from build123d import *

# Parameters (mm, degrees)
RESSALTO_EXTRUS_O1_DEPTH = 56
FILETE1_R                = 0.5
ESBO_O2_R                = 0.751353762
CORTE_EXTRUS_O1_DEPTH    = 57


with BuildPart() as part:
    # Esboço1 → Ressalto-extrusão1 (new body)
    with BuildSketch(Plane.XZ.offset(30)):
        Polygon((-1.443375673, -2.5), (1.443375673, -2.5), (2.886751346, 0), (1.443375673, 2.5), (-1.443375673, 2.5), (-2.886751346, 0), align=None)
    extrude(amount=-RESSALTO_EXTRUS_O1_DEPTH)

    # Filete1
    filete1_edges = [part.edges().sort_by_distance(p)[0] for p in [
        (2.165063509, 26, -1.25),
        (2.165063509, 26, 1.25),
        (0, 26, 2.5),
        (-2.165063509, 26, 1.25),
        (-2.165063509, 26, -1.25),
        (-2.165063509, -30, 1.25),
        (0, -30, 2.5),
        (2.165063509, -30, 1.25),
        (2.165063509, -30, -1.25),
        (0, -30, -2.5),
        (-2.165063509, -30, -1.25),
        (0, 26, -2.5),
    ]]
    fillet(filete1_edges, radius=FILETE1_R)

    # Esboço2 → Corte-extrusão1 (cut, through all)
    with BuildSketch(Plane.XZ.offset(30)):
        Circle(ESBO_O2_R)
    extrude(amount=-CORTE_EXTRUS_O1_DEPTH, mode=Mode.SUBTRACT)


solid = part.part
CAD build for the part. Positions are in the model's coordinates, mm. Round coordinates to 2 decimals unless told otherwise and drop trailing zeros. Loops run counter-clockwise (first coordinate to the right, second up) from the corner with the lowest first, then second, coordinate; pieces in that order, holes last. Notation, with made-up numbers: M 68,27.25 L 90,27.25 A34 ccw 90,58.25 Z; hole C 16,72 d9. An arc over 180 degrees is marked long. One line per question, with ' | ' between items. Start each with the question number.
Item 1: Cut at A-A, the plane y = 21. Write the cut outline in (x, z).
Item 2: Pin check, flat tip, straight feed: pin 1 Ø1 at (y, z) = (-22, 2) entering from +X. Stop position of the tip, or through.
Item 3: Two-plate mould, pull along Z, no slides. Class faces 1 (the flat face through (1, -30, 0)), 2 (the cylindrical face through (-0.098, -2.392, 0.745)), 3 (the cylindrical face through (-2.03, -29.85, -1.2)): pulls with the +Z half, pulls with the -Z half, needs draft (parallel to the pull), parting line crosses it, or undercut.
Item 4: Wall check: line 1 (Z direction, x = 0, y = -17.5); line 2 (X direction, y = 23.5, z = 1); line 3 (Y direction, x = 0.25, z = -2.1). Give the ranges that are in metal, low to high.
Item 5: Cut at B-B, the plane x = 0. Write the cut outline in (y, z), plus the area to 3 significant figures.
Responses:
1) outline: M -2.89,0 L -1.44,-2.5 L 1.44,-2.5 L 2.89,0 L 1.44,2.5 L -1.44,2.5 Z; hole C 0,0 d1.5
2) pin 1: stops at x = 2.02
3) face 1: needs draft | face 2: undercut | face 3: pulls with the -Z half
4) line 1: z = -2.5 to -0.75, 0.75 to 2.5 | line 2: x = -2.31 to 2.31 | line 3: y = -29.99 to 25.99
5) outline: M -30,-2 A0.5 ccw -29.5,-2.5 L 25.5,-2.5 A0.5 ccw 26,-2 L 26,-0.75 L -30,-0.75 Z; M -30,0.75 L 26,0.75 L 26,2 A0.5 ccw 25.5,2.5 L -29.5,2.5 A0.5 ccw -30,2 Z | area: 196 mm²
